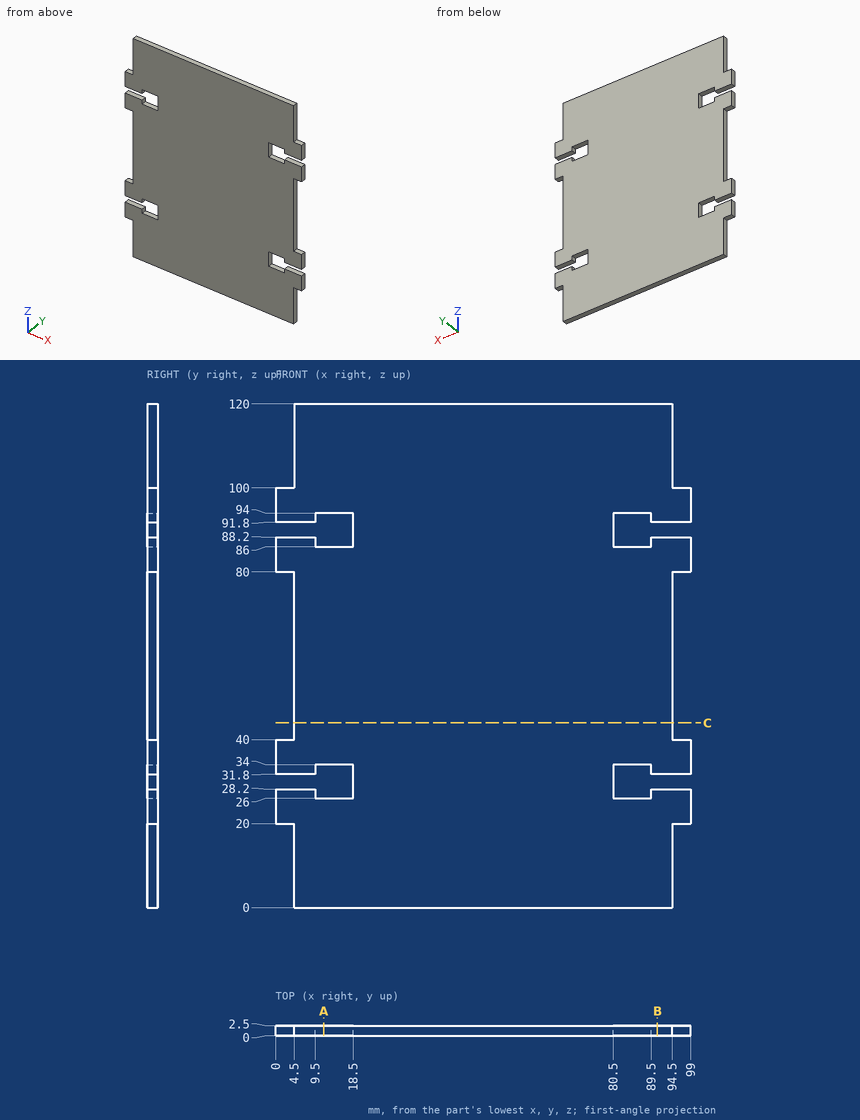
Job drawing, mm, ordinate dimensions from the low corner. One solid piece. Coordinates: 2 decimals unless noted, no trailing zeros. Order: outer loops, then holes, each group sorted by start corner. A loop starts at its lowest first (then second) coordinate and runs counter-clockwise, first axis right, second up. Notation, with made-up numbers: (42.25, 10.25) - (57.25, 10.25) arc R17 cw to (57.25, 32.25) - close; hole circle Ø3 at (4, 25). An arc over 180 degrees is marked (long way). Write each question's results on one line, items separated by ' | '. Start each with the question number.
Item 1: Wall check: probe 1 along X at (y, z) = (1.75, 27.5); probe 2 along Z at (x, y) = (88, 1.1); probe 3 along X at (y, z) = (2.15, 91). Give the ranges that are in metal, low to high. Write a range as [from, to].
Item 2: Flat gauge pins, fed straight in: pin 1 (1.2 mm diameter, centred on x = 2.5, y = 2, fed in from -Z); pin 2 (0.8 mm diameter, centred on y = 1.5, z = 6, fed in from +X); pin 3 (1.2 mm diameter, centred on x = 2, y = 1, fed in from +Z). Where does each tip first touch, or does it go through?
Item 3: Band-saw the part on B-B on x = 91. Write the cut outline in (y, z), and give its area (3 significant figures).
Item 4: Band-saw the part on C-C on z = 44. Write the cut outline in (x, y), and give its area (3 significant figures).
Item 5: Band-saw the part on A-A on x = 11.5. Write the cut outline in (y, z).
Numbers:
1) probe 1: [0, 9.5], [18.5, 80.5], [89.5, 99] | probe 2: [0, 26], [34, 86], [94, 120] | probe 3: [18.5, 80.5]
2) pin 1: z = 20 | pin 2: x = 94.5 | pin 3: z = 100
3) outline: (0, 0) - (2.5, 0) - (2.5, 28.2) - (0, 28.2) - close; (0, 31.8) - (2.5, 31.8) - (2.5, 88.2) - (0, 88.2) - close; (0, 91.8) - (2.5, 91.8) - (2.5, 120) - (0, 120) - close | area: 282 mm^2
4) outline: (4.5, 0) - (94.5, 0) - (94.5, 2.5) - (4.5, 2.5) - close | area: 225 mm^2
5) outline: (0, 0) - (2.5, 0) - (2.5, 26) - (0, 26) - close; (0, 34) - (2.5, 34) - (2.5, 86) - (0, 86) - close; (0, 94) - (2.5, 94) - (2.5, 120) - (0, 120) - close
